from build123d import *

# Parameters (mm, degrees)
SKETCH1_R              = 14.2875
BOSS_EXTRUDE1_DEPTH    = 3.175
SKETCH2_W              = 38.1
SKETCH2_H              = 3.175
BOSS_EXTRUDE2_DEPTH    = 152.4
SKETCH3_R              = 2.45745
CUT_EXTRUDE1_DEPTH     = 195.298586266
CONVERT_SOLID1_START   = -76.2
CONVERT_SOLID1_DEPTH   = 152.4
CONVERT_SOLID1_2_DEPTH = 152.4
SKETCH4_R              = 3.175
CUT_EXTRUDE3_DEPTH     = 198.157018643


# Read off the part's stored shape, not the designer's step: Convert-Solid1
with BuildPart() as part:
    # Sketch1 → Boss-Extrude1 (new body)
    with BuildSketch(Plane(origin=(0, 0, 0), x_dir=(0, 0, -1), z_dir=(1, 0, 0))):
        with BuildLine():
            Line((-76.2, 0), (-76.2, 59.142531573))
            ThreePointArc((-76.2, 59.142531573), (-75.512589628, 63.264144174), (-73.524773161, 66.939577365))
            Line((-73.524773161, 66.939577365), (8.886591171, 172.897045792))
            ThreePointArc((8.886591171, 172.897045792), (13.331600966, 176.508603805), (18.911364332, 177.8))
            Line((18.911364332, 177.8), (63.5, 177.8))
            ThreePointArc((63.5, 177.8), (72.480256121, 174.080256121), (76.2, 165.1))
            Line((76.2, 165.1), (76.2, 0))
            Line((76.2, 0), (-76.2, 0))
        make_face()
        with Locations((38.1, 146.05)):
            Circle(SKETCH1_R, mode=Mode.SUBTRACT)
    extrude(amount=BOSS_EXTRUDE1_DEPTH)

    # Sketch2 → Boss-Extrude2 (add)
    with BuildSketch(Plane.XY.offset(76.2)):
        with Locations((19.05, 1.5875)):
            Rectangle(SKETCH2_W, SKETCH2_H)
    extrude(amount=-BOSS_EXTRUDE2_DEPTH)

    # Sketch3 → Cut-Extrude1 (cut, through all)
    with BuildSketch(Plane(origin=(0, 3.175, 0), x_dir=(1, 0, 0), z_dir=(0, 1, 0))):
        with Locations(Location((19.05, 57.15, 0), (0, 0, 270))):
            Circle(SKETCH3_R)
        with Locations(Location((19.05, 0, 0), (0, 0, 270))):
            Circle(SKETCH3_R)
        with Locations(Location((19.05, -57.15, 0), (0, 0, 270))):
            Circle(SKETCH3_R)
    extrude(amount=-CUT_EXTRUDE1_DEPTH, mode=Mode.SUBTRACT)

    # Convert-Solid1 outline → Convert-Solid1 (cut)
    with BuildSketch(Plane.XY.offset(CONVERT_SOLID1_START)):
        with BuildLine():
            Line((0, 0), (4.445, 0))
            ThreePointArc((4.445, 0), (1.301910358, 1.301910358), (0, 4.445))
            Line((0, 4.445), (0, 0))
        make_face()
    extrude(amount=CONVERT_SOLID1_DEPTH, mode=Mode.SUBTRACT)

    # Convert-Solid1 2 outline → Convert-Solid1 2 (add)
    with BuildSketch(Plane.XY.offset(CONVERT_SOLID1_START)):
        with BuildLine():
            Line((3.175, 3.175), (4.445, 3.175))
            ThreePointArc((4.445, 3.175), (3.546974388, 3.546974388), (3.175, 4.445))
            Line((3.175, 4.445), (3.175, 3.175))
        make_face()
    extrude(amount=CONVERT_SOLID1_2_DEPTH)

    # Sketch4 → Cut-Extrude3 (cut, through all)
    with BuildSketch(Plane.ZY):
        with Locations((50.8, 50.8)):
            Circle(SKETCH4_R)
    extrude(amount=-CUT_EXTRUDE3_DEPTH, mode=Mode.SUBTRACT)


solid = part.part
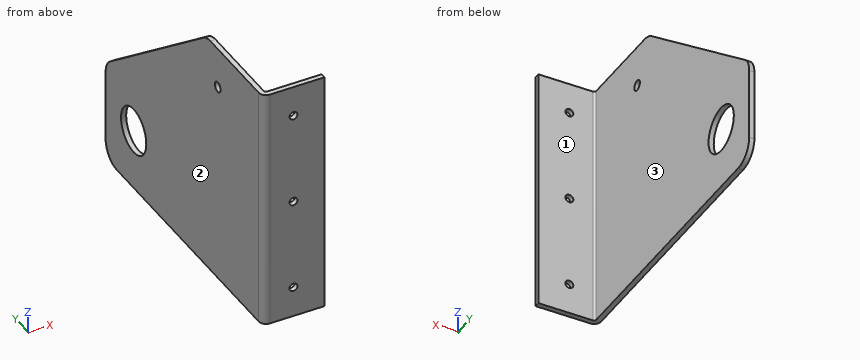
Input: part model. Units: mm. Frame: model coordinates. Face numbers are marked on the shaded views. Coordinates: 2 decimals unless noted, no trailing zeros. Order: outer loops, then holes, each group sorted by start corner. A loop starts at its lowest first (then second) coordinate and runs counter-clockwise, first axis right, second up. Notation, with made-up numbers: M 1.5,-12 L 39.5,-12 A20 ccw 39.5,-5 Z; hole C -19,75.5 d10. An arc over 180 degrees is marked long. Answer as CSV lines item,"result".
1. Section D-D (z = 50.8). Return the cut outline in (x, y) (3 decimals), then the cut area to 3 significant figures.
Reported:
outline,"M 0,4.445 A4.445 ccw 4.445,0 L 38.1,0 L 38.1,3.175 L 4.445,3.175 A1.27 cw 3.175,4.445 L 3.175,47.625 L 0,47.625 Z; M 0,53.975 L 3.175,53.975 L 3.175,96.157 L 0,96.157 Z"
area,"392 mm2"
2. Section C-C (z = -57.15). Return the cut outline in (x, y) (3 decimals).
Reported:
outline,"M 0,4.445 A4.445 ccw 4.445,0 L 16.593,0 L 16.593,3.175 L 4.445,3.175 A1.27 cw 3.175,4.445 L 3.175,177.8 L 0,177.8 Z; M 21.507,0 L 38.1,0 L 38.1,3.175 L 21.507,3.175 Z"
3. Section B-B (y = 146.05). Return the cut outline in (x, z) (1 decimal).
Reported:
outline,"M 0,-76.2 L 3.2,-76.2 L 3.2,-52.4 L 0,-52.4 Z; M 0,-23.8 L 3.2,-23.8 L 3.2,12 L 0,12 Z"
4. Material intervals for line 1 (Z direction, x = 19, y = 1); line 2 (X direction, y = 105.5, z = -15) (3 decimals), sorted ascending. Write a range as from..to.
Reported:
line 1,"-76.2..-59.61, -54.69..-2.46, 2.46..54.69, 59.61..76.2"
line 2,"0..3.175"
5. Section A-A (x = 19.05). Return the cut outline in (y, z) (3 decimals), then the cut area to 3 significant figures.
Reported:
outline,"M 0,-76.2 L 3.175,-76.2 L 3.175,-59.607 L 0,-59.607 Z; M 0,-54.693 L 3.175,-54.693 L 3.175,-2.457 L 0,-2.457 Z; M 0,2.457 L 3.175,2.457 L 3.175,54.693 L 0,54.693 Z; M 0,59.607 L 3.175,59.607 L 3.175,76.2 L 0,76.2 Z"
area,"437 mm2"
6. Pull-direction query (X, two-part tool) for the marked faces 1, 2 and 3; classes: released by +X, released by -X, zero draft, split by the parting line, or undercut.
Reported:
face 1,"zero draft"
face 2,"released by -X"
face 3,"released by +X"
7. First-contact query: P1, Ø8, axis at y = 63, z = 8.5, coming from the +X side (3 decimals); P2, Ø5.5, axis at x = 19.05, z = 0, coming from the +Y side (3 decimals); P3, Ø5.5, axis at y = 50.8, z = 50.8, coming from the +X side; P4, Ø5, axis at x = 5.5, y = 115, coming from the +Z side. Flat tips, straight axial feed; report the tip coordinate or a pass-through.
Reported:
P1,"x = 3.175"
P2,"y = 3.175"
P3,"through"
P4,"z = 36.86"
